Could you check a few things on this model? Use its own coordinates, in mm. Face numbers are marked on the shaded views. A direction names the side the tool comes from. Give positions to 0.01 mm unless a question says otherwise; leave off trailing zeros. Loops run counter-clockwise (first coordinate to the right, second up) from the corner with the lowest first, then second, coordinate; pieces in that order, holes last. Notation, with made-up numbers: M 60.25,33 L 119.25,33 A30 cw 119.25,60 Z; hole C 60,11 d3. An arc over 180 degrees is marked long. Use a Markdown table: item, result. Add a question column.
1) Suppose I cut it at A-A on z = 5.5. List the corners of the cut face in (x, y) for me.
2) Will these pins go through, and if not, where does the flat tip stop? pin 1 Ø7.5 at (x, y) = (-1, 3) entering from +Z; pin 2 Ø3 at (x, y) = (0, -1) entering from -Z (3 decimals); pin 3 Ø8 at (x, z) = (4.5, 0) entering from +Y; pin 4 Ø1 at (y, z) = (-5.5, 3.5) entering from -X.
3) If I drill on line 1 along Y through (x, z) = (0, -11.8); line 2 along Y through (x, z) = (0, 3); line 3 along Z through (x, y) = (1, 6), over which ranges is the centre line in solid material (lowest first)? Write a range as [from, to].
4) We'd pull the mould along Y, two halves only. Please class the marked faces 4 and 5: +Y half, -Y half, draft (parallel to the pull), parting line (faces both ways), or undercut.
5) Which directions (+Z, -Z, +X, -X, +Y, -Y) give clear straight access to the entire face, cutting with the end or side of a thin tool? Please do the marked faces 1, 2 and 3.
```python
from build123d import *

# Parameters (mm, degrees)
ESBO_O1_R                = 7.5
ESBO_O1_R_2              = 4
RESSALTO_EXTRUS_O1_DEPTH = 12
ESBO_O2_R                = 6.5
ESBO_O2_R_2              = 4.5
CORTE_EXTRUS_O1_DEPTH    = 0.5
CORTE_EXTRUS_O2_START    = -0.5
ESBO_O3_R                = 6.5
ESBO_O3_R_2              = 4.5
CORTE_EXTRUS_O2_DEPTH    = 0.5
ESBO_O4_R                = 8.150175923
ESBO_O4_R_2              = 7.3
CORTE_EXTRUS_O3_DEPTH    = 0.2
FILETE1_R                = 0.25


with BuildPart() as part:
    # Esboço1 → Ressalto-extrusão1 (new, symmetric)
    with BuildSketch(Plane.XY):
        Circle(ESBO_O1_R)
        Circle(ESBO_O1_R_2, mode=Mode.SUBTRACT)
    extrude(amount=RESSALTO_EXTRUS_O1_DEPTH, both=True)

    # Esboço2 → Corte-extrusão1 (cut)
    with BuildSketch(Plane.XY.offset(12)):
        Circle(ESBO_O2_R)
        Circle(ESBO_O2_R_2, mode=Mode.SUBTRACT)
    extrude(amount=-CORTE_EXTRUS_O1_DEPTH, mode=Mode.SUBTRACT)

    # Esboço3 → Corte-extrusão2 (cut)
    with BuildSketch(Plane(origin=(0, 0, -12), x_dir=(-1, 0, 0), z_dir=(0, 0, -1)).offset(CORTE_EXTRUS_O2_START)):
        with Locations(Location((0, 0, 0), (0, 0, 180))):
            Circle(ESBO_O3_R)
        with Locations(Location((0, 0, 0), (0, 0, 180))):
            Circle(ESBO_O3_R_2, mode=Mode.SUBTRACT)
    extrude(amount=CORTE_EXTRUS_O2_DEPTH, mode=Mode.SUBTRACT)

    # Esboço4 → Corte-extrusão3 (cut)
    with BuildSketch(Plane.XY.offset(8)):
        Circle(ESBO_O4_R)
        Circle(ESBO_O4_R_2, mode=Mode.SUBTRACT)
    corte_extrus_o3 = extrude(amount=CORTE_EXTRUS_O3_DEPTH, mode=Mode.SUBTRACT)

    # Espelhar1: Corte-extrusão3 across plane
    add(corte_extrus_o3.mirror(Plane.XY), mode=Mode.SUBTRACT)

    # Filete1
    filete1_edges = [part.edges().sort_by_distance(p)[0] for p in [
        (-7.5, 0, -12),
        (-7.5, 0, 12),
    ]]
    fillet(filete1_edges, radius=FILETE1_R)


solid = part.part
```
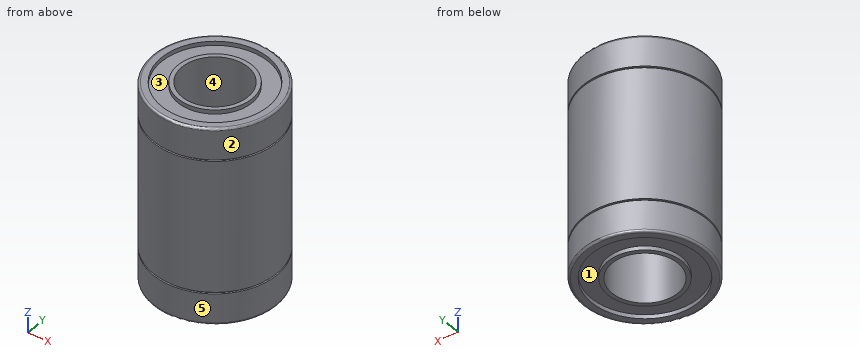
Answer block:
| question | item | result |
|---|---|---|
| 1 | outline | C 0,0 d15; hole C 0,0 d8 |
| 2 | pin 1 | stops at z = 12 |
| 2 | pin 2 | passes through |
| 2 | pin 3 | stops at y = 7.48 |
| 2 | pin 4 | stops at x = -5.59 |
| 3 | line 1 | y = [-7.49, -6.5], [-4.5, -4], [4, 4.5], [6.5, 7.49] |
| 3 | line 2 | y = [-7.5, -4], [4, 7.5] |
| 3 | line 3 | z = [-11.5, 11.5] |
| 4 | face 4 | undercut |
| 4 | face 5 | parting line |
| 5 | face 1 | -Z |
| 5 | face 2 | +Z, -Z |
| 5 | face 3 | +Z |
